```python
from build123d import *

# Parameters (mm, degrees)
SKETCH1_W           = 30.4
SKETCH1_H           = 42
BOSS_EXTRUDE1_DEPTH = 5
SKETCH2_W           = 42
SKETCH2_H           = 3.2
BOSS_EXTRUDE2_DEPTH = 8.49
SKETCH4_W           = 30.4
SKETCH4_H           = 1.4
BOSS_EXTRUDE3_DEPTH = 20
SKETCH5_R           = 3.875
SKETCH5_R_2         = 1
CUT_EXTRUDE1_DEPTH  = 1.4
CHAMFER1_SIZE       = 4.5
SKETCH6_R           = 1.5
CUT_EXTRUDE2_DEPTH  = 5
SKETCH7_W           = 38.89
SKETCH7_H           = 2
BOSS_EXTRUDE4_DEPTH = 12.5
SKETCH8_R           = 10.4
CUT_EXTRUDE3_DEPTH  = 2


with BuildPart() as part:
    # Sketch1 → Boss-Extrude1 (new body)
    with BuildSketch(Plane(origin=(0, 0, 0), x_dir=(1, 0, 0), z_dir=(0, 1, 0))):
        Rectangle(SKETCH1_W, SKETCH1_H)
    extrude(amount=BOSS_EXTRUDE1_DEPTH)

    # Sketch2 → Boss-Extrude2 (add)
    with BuildSketch(Plane.ZY.offset(15.2)):
        with Locations((0, 3.4)):
            Rectangle(SKETCH2_W, SKETCH2_H)
    extrude(amount=BOSS_EXTRUDE2_DEPTH)

    # Sketch4 → Boss-Extrude3 (add)
    with BuildSketch(Plane(origin=(0, 5, 0), x_dir=(1, 0, 0), z_dir=(0, 1, 0))):
        with Locations((-8.49, -20.3)):
            Rectangle(SKETCH4_W, SKETCH4_H)
    extrude(amount=BOSS_EXTRUDE3_DEPTH)

    # Sketch5 → Cut-Extrude1 (cut)
    with BuildSketch(Plane(origin=(0, 0, 19.6), x_dir=(-1, 0, 0), z_dir=(0, 0, -1))):
        with Locations((8.49, 17.78)):
            Circle(SKETCH5_R)
        with Locations((0.74, 17.78)):
            Circle(SKETCH5_R_2)
        with Locations((16.24, 17.78)):
            Circle(SKETCH5_R_2)
    extrude(amount=-CUT_EXTRUDE1_DEPTH, mode=Mode.SUBTRACT)

    # Chamfer1
    chamfer1_edges = [part.edges().sort_by_distance(p)[0] for p in [
        (-23.69, 25, 20.3),
        (6.71, 25, 20.3),
    ]]
    chamfer(chamfer1_edges, length=CHAMFER1_SIZE)

    # Sketch6 → Cut-Extrude2 (cut)
    with BuildSketch(Plane(origin=(0, 5, 0), x_dir=(1, 0, 0), z_dir=(0, 1, 0))):
        with Locations(Location((12.5, -15.6, 0), (0, 0, 270))):
            Circle(SKETCH6_R)
        with Locations(Location((12.5, 17, 0), (0, 0, 270))):
            Circle(SKETCH6_R)
        with Locations(Location((-12.5, 17, 0), (0, 0, 270))):
            Circle(SKETCH6_R)
        with Locations(Location((-12.5, -15.6, 0), (0, 0, 270))):
            Circle(SKETCH6_R)
    extrude(amount=-CUT_EXTRUDE2_DEPTH, mode=Mode.SUBTRACT)

    # Sketch7 → Boss-Extrude4 (add)
    with BuildSketch(Plane(origin=(0, 5, 0), x_dir=(1, 0, 0), z_dir=(0, 1, 0))):
        with Locations((-4.245, 7.28)):
            Rectangle(SKETCH7_W, SKETCH7_H)
    extrude(amount=BOSS_EXTRUDE4_DEPTH)

    # Sketch8 → Cut-Extrude3 (cut)
    with BuildSketch(Plane(origin=(0, 0, -8.28), x_dir=(-1, 0, 0), z_dir=(0, 0, -1))):
        with Locations((8.49, 17.5)):
            Circle(SKETCH8_R)
    extrude(amount=-CUT_EXTRUDE3_DEPTH, mode=Mode.SUBTRACT)


solid = part.part
```
Check sheet for the modelled part. Datum: model origin and axes. Units: mm. A direction names the side the tool comes from. Give positions to 0.01 mm unless a question says otherwise; leave off trailing zeros. Write each loop counter-clockwise with the first axis right and the second up, starting at its lowest first coordinate (ties: lowest second). Pieces come first, ordered by that corner, then holes. Notation, with made-up numbers: (22, -20) - (46, -20) arc R34 ccw to (46, 18) - close; hole circle Ø1 at (11.25, -15.75). An arc over 180 degrees is marked (long way). Answer as a JSON object with one key per item and string values. Group by question number.
1) Depth check by flat-ended pin: P1, Ø7, axis at x = -20.5, z = -5, coming from the -Y side; P2, Ø2, axis at x = -7.5, y = 13.5, coming from the -Z side; P3, Ø0.7, axis at y = 10.5, z = 20.5, coming from the +X side; P4, Ø1.6, axis at x = -0.74, y = 17.78, coming from the +Z side. Enter the tip coordinate at first touch or a pass-through.
2) Thickness scan on probe 1 along X at (y, z) = (3.1, -17); probe 2 along Z at (x, y) = (0, 10); probe 3 along Y at (x, z) = (-0.74, 20.2). Record the ranges inside material, lowest first. Write a range as from..to.
3) Sectioned sample at D-D (x = 5.5). Record the cut outline in (y, z).
4) Sectioned sample at B-B (z = 15.6). Record the cut outline in (x, y), then the cut area to 3 significant figures.
5) Release check for a two-part mould opening along Z. For faces 4 (the face through (-9, 12, 21)), 5 (the face through (-4, 5, 7)), 6 (the face through (0, 10, -8.28)) record: pulls with the +Z half, pulls with the -Z half, needs draft (parallel to the pull), parting line crosses it, or undercut.
6) Sectioned sample at A-A (x = 12.5). Record the cut outline in (y, z).
7) Access from +Z, -Z, +X, -X, +Y, -Y to the whole of each face (thin tool, end or side, straight path). Record for faces 1 (the face through (6.71, 13, 20)), 2 (the face through (-4, 5, -15)), 3 (the face through (-19, 1.8, 0)).
8) Sectioned sample at C-C (y = 10.5). Record the cut outline in (x, z), then the cut area to 3 significant figures.
Geometry results:
{
 "1": {"P1": "stops at y = 1.8", "P2": "stops at z = 19.6", "P3": "stops at x = 6.71", "P4": "passes through"},
 "2": {"probe 1": "x = -23.69..-14, -11..11, 14..15.2", "probe 2": "z = -8.28..-6.28, 19.6..21", "probe 3": "y = 0..16.78, 18.78..25"},
 "3": {"outline": "(0, -21) - (5, -21) - (5, -8.28) - (17.5, -8.28) - (17.5, -6.28) - (5, -6.28) - (5, 19.6) - (21.71, 19.6) - (21.71, 21) - (0, 21) - close"},
 "4": {"outline": "(-23.69, 1.8) - (-15.2, 1.8) - (-15.2, 0) - (-14, 0) - (-14, 5) - (-23.69, 5) - close; (-11, 0) - (11, 0) - (11, 5) - (-11, 5) - close; (14, 0) - (15.2, 0) - (15.2, 5) - (14, 5) - close", "area": "149 mm^2"},
 "5": {"face 4": "pulls with the +Z half", "face 5": "undercut", "face 6": "pulls with the -Z half"},
 "6": {"outline": "(0, -21) - (5, -21) - (5, -18.5) - (0, -18.5) - close; (0, -15.5) - (5, -15.5) - (5, -8.28) - (17.5, -8.28) - (17.5, -6.28) - (5, -6.28) - (5, 14.1) - (0, 14.1) - close; (0, 17.1) - (5, 17.1) - (5, 21) - (0, 21) - close"},
 "7": {"face 1": "+Z, +X, +Y", "face 2": "-Z, +X, -X, +Y", "face 3": "+Z, -Z, -X, -Y"},
 "8": {"outline": "(-23.69, -8.28) - (-16.18, -8.28) - (-16.18, -6.28) - (-23.69, -6.28) - close; (-23.69, 19.6) - (6.71, 19.6) - (6.71, 21) - (-23.69, 21) - close; (-0.8, -8.28) - (15.2, -8.28) - (15.2, -6.28) - (-0.8, -6.28) - close", "area": "89.6 mm^2"}
}
